Model file for the job. Use its own axes, mm. A direction names the side the tool comes from. Coordinates: 2 decimals unless noted, no trailing zeros. Order: outer loops, then holes, each group sorted by start corner. A loop starts at its lowest first (then second) coordinate and runs counter-clockwise, first axis right, second up. Notation, with made-up numbers: M 41,-24 L 67,-24 A22 cw 67,-9 Z; hole C 53.5,75.25 d4. An arc over 180 degrees is marked long. Return JSON: item names as keys, results as strings.
```python
from build123d import *

# Parameters (mm, degrees)
F1_DEPTH = 1.5
F3_DEPTH = 7
F4_R     = 1.5
F5_DEPTH = 7.001
F6_R     = 2
F7_DEPTH = 5.001
F9_DEPTH = 7.001


with BuildPart() as f1:
    # F0 (on Top) → F1 (new body, symmetric)
    with BuildSketch(Plane.XY):
        Polygon((-1.090006, 3.5), (-3.090006, 1.5), (-3.090006, -1.5), (-1.090006, -3.5), (12.909994, -3.5), (12.909994, 3.5), align=None)
    extrude(amount=F1_DEPTH, both=True)

    # F2 (on face) → F3 (join)
    with BuildSketch(Plane.XZ.offset(3.5)):
        Polygon((6.909994, 3.5), (4.909994, 1.5), (12.909994, 1.5), (12.909994, 3.5), align=None)
        Polygon((12.909994, -1.5), (4.909994, -1.5), (6.909994, -3.5), (12.909994, -3.5), align=None)
    extrude(amount=-F3_DEPTH)

    # F4 (on face) → F5 (cut, through all)
    with BuildSketch(Plane.XZ.offset(3.5)):
        with Locations((9.409994, 0)):
            Circle(F4_R)
    extrude(amount=-F5_DEPTH, mode=Mode.SUBTRACT)

    # F6 (on face) → F7 (cut, through all)
    with BuildSketch(Plane.XY.offset(1.5)):
        with Locations((0.909994, 0)):
            Circle(F6_R)
    extrude(amount=-F7_DEPTH, mode=Mode.SUBTRACT)

    # F8 (on face) → F9 (cut, through all)
    with BuildSketch(Plane.XZ.offset(3.5)):
        with BuildLine():
            ThreePointArc((9.409994, 3.5), (11.884868, 2.474874), (12.909994, 0))
            Line((12.909994, 0), (12.909994, 3.5))
            Line((12.909994, 3.5), (9.409994, 3.5))
        make_face()
        with BuildLine():
            ThreePointArc((12.909994, 0), (11.884868, -2.474874), (9.409994, -3.5))
            Line((9.409994, -3.5), (12.909994, -3.5))
            Line((12.909994, -3.5), (12.909994, 0))
        make_face()
    extrude(amount=-F9_DEPTH, mode=Mode.SUBTRACT)


solid = f1.part
```
Item 1: Saw through at B-B (z = 1.25). Write the cut outline in (x, y).
Check result:
{"outline": "M -3.09,-1.5 L -1.09,-3.5 L 8.58,-3.5 L 8.58,3.5 L -1.09,3.5 L -3.09,1.5 Z; M 10.24,-3.5 L 12.68,-3.5 L 12.68,3.5 L 10.24,3.5 Z; hole C 0.91,0 d4"}
Item 2: 3-axis set-ups, long thin cutter, end or side, ignore diameter. For faces 4 (the flat face through (3, 2, 1.5)), 5 (the flat face through (8, 0, -3.5)): which of +Z, -Z, +X, -X, +Y, -Y reach the whole face in a straight line?
Check result:
{"face 4": "+Z, -X, +Y, -Y", "face 5": "-Z, +X, -X, +Y, -Y"}
Item 3: Wall check: line 1 (Z direction, x = -1.5, y = 0.75); line 2 (Z direction, x = 9.5, y = -2.25); line 3 (X direction, y = 3, z = 0.5). Give the ranges that are in metal, low to high.
Check result:
{"line 1": "z = -1.5 to 1.5", "line 2": "z = -3.5 to -1.5, 1.5 to 3.5", "line 3": "x = -1.59 to 8, 10.82 to 12.87"}
Item 4: Saw through at D-D (x = 10). Write the cut outline in (y, z), and give its area (3 significant figures).
Check result:
{"outline": "M -3.5,-3.45 L 3.5,-3.45 L 3.5,-1.38 L -3.5,-1.38 Z; M -3.5,1.38 L 3.5,1.38 L 3.5,3.45 L -3.5,3.45 Z", "area": "29.0 mm2"}
Item 5: Saw through at A-A (y = 0). Write the cut outline in (x, z).
Check result:
{"outline": "M -3.09,-1.5 L -1.09,-1.5 L -1.09,1.5 L -3.09,1.5 Z; M 2.91,-1.5 L 4.91,-1.5 L 6.91,-3.5 L 9.41,-3.5 A3.5 ccw 12.91,0 A3.5 ccw 9.41,3.5 L 6.91,3.5 L 4.91,1.5 L 2.91,1.5 Z; hole C 9.41,0 d3"}
Item 6: Saw through at C-C (y = 2.5). Write the cut outline in (x, z).
Check result:
{"outline": "M -2.09,-1.5 L 4.91,-1.5 L 6.91,-3.5 L 9.41,-3.5 A3.5 ccw 12.91,0 A3.5 ccw 9.41,3.5 L 6.91,3.5 L 4.91,1.5 L -2.09,1.5 Z; hole C 9.41,0 d3"}
Item 7: Drop flat-ended pins along their axis: pin 1 Ø3 at (y, z) = (-0.5, -2.5) entering from +X; pin 2 Ø2 at (x, y) = (0, -1.5) entering from +Z. Give the stop position or say it passes through.
Check result:
{"pin 1": "stops at x = 12.76", "pin 2": "stops at z = 1.5"}
Item 8: Pull direction Z, two halves, no side cores. Call faces 1 (the flat face through (-3.09, 0, 0)), 2 (the flat face through (3, 2, -1.5)), 3 (the cylindrical face through (8.22, -0.05, -0.91)): +Z half, -Z half, draft (parallel to the pull), parting line (faces both ways), or undercut.
Check result:
{"face 1": "draft", "face 2": "-Z half", "face 3": "undercut"}
